Model file for the job. Use its own axes, mm. A direction names the side the tool comes from. Give positions to 0.01 mm unless a question says otherwise; leave off trailing zeros. Loops run counter-clockwise (first coordinate to the right, second up) from the corner with the lowest first, then second, coordinate; pieces in that order, holes last. Notation, with made-up numbers: M 71,56 L 79,56 A30 cw 79,79 Z; hole C -26,8.25 d9. An arc over 180 degrees is marked long. Answer in a Markdown table with one row per item.
```python
from build123d import *

# Parameters (mm, degrees)
F1_DEPTH = 1030
F2_R     = 17.5
F2_R_2   = 15
F3_DEPTH = 55
F4_R     = 17.5
F4_R_2   = 15
F5_DEPTH = 55


with BuildPart() as f1:
    # F0 (on Front) → F1 (new body)
    with BuildSketch(Plane.XZ):
        with BuildLine():
            Line((5.830952, 16.5), (-5.830952, 16.5))
            ThreePointArc((-5.830952, 16.5), (0, -17.5), (5.830952, 16.5))
        make_face()
    extrude(amount=F1_DEPTH)

    # F2 (on Front) → F3 (cut)
    with BuildSketch(Plane.XZ):
        Circle(F2_R)
        Circle(F2_R_2, mode=Mode.SUBTRACT)
    extrude(amount=F3_DEPTH, mode=Mode.SUBTRACT)

    # F4 (on face) → F5 (cut)
    with BuildSketch(Plane.XZ.offset(1030)):
        Circle(F4_R)
        Circle(F4_R_2, mode=Mode.SUBTRACT)
    extrude(amount=-F5_DEPTH, mode=Mode.SUBTRACT)


solid = f1.part
```
(1) Flat gauge pins, fed straight in: P1, Ø10, axis at x = -13.5, y = -386, coming from the +Z side; P2, Ø2, axis at x = 5, y = -716, coming from the -Z side; P3, Ø3, axis at x = 11, y = -569, coming from the -Z side. Where does each tip first touch, or does it go through?
Established:
| item | result |
|---|---|
| P1 | stops at z = 15.3 |
| P2 | stops at z = -17.04 |
| P3 | stops at z = -14.7 |
(2) Saw through at B-B, the plane y = -690. Give the cut face in (x, z), and give its area (3 significant figures).
Established:
| item | result |
|---|---|
| outline | M -5.83,16.5 A17.5 ccw long 5.83,16.5 Z |
| area | 954 mm2 |
(3) Which spindle directions (+Z, -Z, +X, -X, +Y, -Y) get a long thin tool onto all of the face, cutting with end or side? Do faces 1 (the cylindrical face through (-0.686, -508.56, -17.487)), 2 (the flat face through (5.1, -55, -14.3)), 3 (the cylindrical face through (-14.985, -1002.885, 0.66)). Say none if no direction does.
Established:
| item | result |
|---|---|
| face 1 | +Y, -Y |
| face 2 | +Y |
| face 3 | -Y |
(4) Wall check: L1, parallel to Z at x = -2, y = -923; L2, parallel to X at y = -200.5, z = -2; L3, parallel to Y at x = 16, z = -5.5. Give the ranges that are in metal, low to high.
Established:
| item | result |
|---|---|
| L1 | z = -17.39 to 16.5 |
| L2 | x = -17.39 to 17.39 |
| L3 | y = -975 to -55 |
(5) Saw through at A-A, the plane z = 0. Give the cut face in (x, y).
Established:
| item | result |
|---|---|
| outline | M -17.5,-975 L -15,-975 L -15,-1030 L 15,-1030 L 15,-975 L 17.5,-975 L 17.5,-55 L 15,-55 L 15,0 L -15,0 L -15,-55 L -17.5,-55 Z |
